Could you check a few things on this model? Use its own coordinates, in mm. Face numbers are marked on the shaded views. A direction names the side the tool comes from. Give positions to 0.01 mm unless a question says otherwise; leave off trailing zeros. Order: outer loops, then holes, each group sorted by start corner. A loop starts at its lowest first (then second) coordinate and runs counter-clockwise, first axis right, second up.
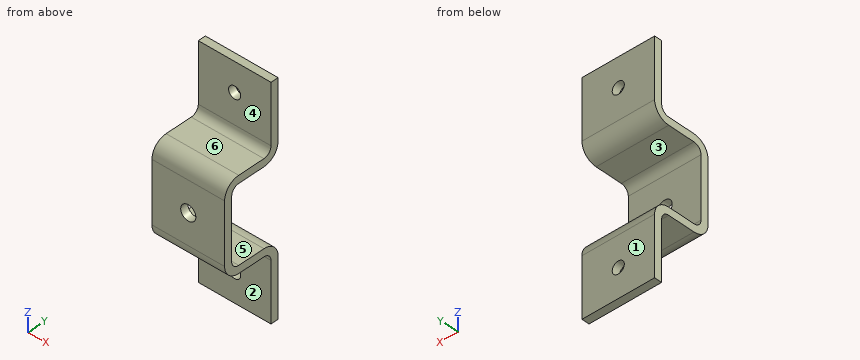
from build123d import *

# Parameters (mm, degrees)
BOSS_EXTRUDE3_START = -76.2
BOSS_EXTRUDE3_DEPTH = 76.2
SKETCH3_R           = 7.9375
CUT_EXTRUDE1_DEPTH  = 76.2
SKETCH2_R           = 6.35
CUT_EXTRUDE3_DEPTH  = 76.2


# Read off the part's stored shape, not the designer's step: Boss-Extrude3
with BuildPart() as part:
    # Boss-Extrude3 outline → Boss-Extrude3 (new body)
    with BuildSketch(Plane.YZ.offset(BOSS_EXTRUDE3_START)):
        with BuildLine():
            Line((44.228000004, 47.750520151), (15.875, 47.750520151))
            ThreePointArc((15.875, 47.750520151), (4.649679848, 43.100840303), (0, 31.875520151))
            Line((0, 31.875520151), (0, -31.875520151))
            ThreePointArc((0, -31.875520151), (4.649679849, -43.100840302), (15.875, -47.750520151))
            Line((15.875, -47.750520151), (44.228000004, -47.750520151))
            ThreePointArc((44.228000004, -47.750520151), (49.849640336, -50.079079819), (52.178200004, -55.700720151))
            Line((52.178200004, -55.700720151), (52.178200004, -117.475))
            Line((52.178200004, -117.475), (60.128400004, -117.475))
            Line((60.128400004, -117.475), (60.128400004, -55.675320151))
            ThreePointArc((60.128400004, -55.675320151), (55.478720155, -44.45), (44.253400004, -39.800320151))
            Line((44.253400004, -39.800320151), (15.9004, -39.800320151))
            ThreePointArc((15.9004, -39.800320151), (10.278759668, -37.471760483), (7.9502, -31.850120151))
            Line((7.9502, -31.850120151), (7.9502, 31.850120151))
            ThreePointArc((7.9502, 31.850120151), (10.278759668, 37.471760483), (15.9004, 39.800320151))
            Line((15.9004, 39.800320151), (44.253400004, 39.800320151))
            ThreePointArc((44.253400004, 39.800320151), (55.478720155, 44.45), (60.128400004, 55.675320151))
            Line((60.128400004, 55.675320151), (60.128400004, 117.475))
            Line((60.128400004, 117.475), (52.178200004, 117.475))
            Line((52.178200004, 117.475), (52.178200004, 55.700720151))
            ThreePointArc((52.178200004, 55.700720151), (49.849640335, 50.079079819), (44.228000004, 47.750520151))
        make_face()
    extrude(amount=BOSS_EXTRUDE3_DEPTH)

    # Sketch3 → Cut-Extrude1 (cut)
    with BuildSketch(Plane(origin=(0, 7.9502, 0), x_dir=(1, 0, 0), z_dir=(0, 1, 0))):
        with Locations(Location((-38.1, 0, 0), (0, 0, 270))):
            Circle(SKETCH3_R)
    extrude(amount=-CUT_EXTRUDE1_DEPTH, mode=Mode.SUBTRACT)

    # Sketch2 → Cut-Extrude3 (cut)
    with BuildSketch(Plane(origin=(0, 60.128400004, 0), x_dir=(1, 0, 0), z_dir=(0, 1, 0))):
        with Locations(Location((-38.1, 87.2998, 0), (0, 0, 270))):
            Circle(SKETCH2_R)
        with Locations(Location((-38.1, -87.2998, 0), (0, 0, 270))):
            Circle(SKETCH2_R)
    extrude(amount=-CUT_EXTRUDE3_DEPTH, mode=Mode.SUBTRACT)


solid = part.part
Item 1: Imagine slicing it at A-A on x = -38.1. Give the number of separate pieces and of enclosed holes in the cut face, then the cut area to 3 significant figures.
Findings:
separate pieces: 4
enclosed holes: 0
area: 2,210 mm2
Item 2: Imagine slicing it at D-D on x = -7. List the corners of the cut face in (y, z) for me (3 decimals), then the cut area to 3 significant figures.
Findings:
outline: (0, -31.876) arc R15.875 ccw to (15.875, -47.751) - (44.228, -47.751) arc R7.95 cw to (52.178, -55.701) - (52.178, -117.475) - (60.128, -117.475) - (60.128, -55.675) arc R15.875 ccw to (44.253, -39.8) - (15.9, -39.8) arc R7.95 cw to (7.95, -31.85) - (7.95, 31.85) arc R7.95 cw to (15.9, 39.8) - (44.253, 39.8) arc R15.875 ccw to (60.128, 55.675) - (60.128, 117.475) - (52.178, 117.475) - (52.178, 55.701) arc R7.95 cw to (44.228, 47.751) - (15.875, 47.751) arc R15.875 ccw to (0, 31.876) - close
area: 2,540 mm2
Item 3: Imagine slicing it at C-C on y = 30. List the corners of the cut face in (x, z) for me, then the cut area to 3 significant figures.
Findings:
outline: (-76.2, -47.75) - (0, -47.75) - (0, -39.8) - (-76.2, -39.8) - close; (-76.2, 39.8) - (0, 39.8) - (0, 47.75) - (-76.2, 47.75) - close
area: 1,210 mm2
Item 4: For pin 1 (8.5 mm diameter, centred on x = -39.5, y = 33, fed in from +Z); pin 2 (4 mm diameter, centred on x = -43.5, y = 35.5, fed in from -Z); pin 3 (1 mm diameter, centred on x = -23.5, z = -12.5, fed in from +Y); pin 4 (12.5 mm diameter, centred on x = -38.1, z = 0, fed in from -Y), each with a flat end and sliding along its axis, tell me the tip position at first contact or that it passes through.
Findings:
pin 1: stops at z = 47.75
pin 2: stops at z = -47.75
pin 3: stops at y = 7.95
pin 4: passes through
Item 5: We'd pull the mould along Z, two halves only. Please class the marked faces 4, 5 and 6: +Z half, -Z half, draft (parallel to the pull), parting line (faces both ways), or undercut.
Findings:
face 4: draft
face 5: undercut
face 6: +Z half
Item 6: For the marked faces 1, 2 and 3, which set-ups out of +Z, -Z, +X, -X, +Y, -Y let a thin tool reach every point of the face, with its end or its side?
Findings:
face 1: +Z, -Z, +X, -X, +Y
face 2: -Z, +X, -X, -Y
face 3: +X, -X, +Y
Item 7: Imagine slicing it at B-B on z = 0. List the corners of the cut face in (x, y) for me.
Findings:
outline: (-76.2, 0) - (-46.04, 0) - (-46.04, 7.95) - (-76.2, 7.95) - close; (-30.16, 0) - (0, 0) - (0, 7.95) - (-30.16, 7.95) - close
Item 8: Please list where these lines run through material, in increasing order: line 1 along X through (y, z) = (4.5, 0); line 2 along Z through (x, y) = (-30, 44); line 3 along Y through (x, z) = (-55, 87.5).
Findings:
line 1: x = -76.2 to -46.04, -30.16 to 0
line 2: z = -47.75 to -39.8, 39.8 to 47.75
line 3: y = 52.18 to 60.13
